Could you check a few things on this model? Use its own coordinates, in mm. Give positions to 0.01 mm unless a question says otherwise; leave off trailing zeros. Write each loop counter-clockwise with the first axis right and the second up, starting at its lowest first coordinate (ties: lowest second). Pieces come first, ordered by that corner, then holes. Notation, with made-up numbers: M 47,38.25 L 67,38.25 A20 cw 67,64.25 Z; hole C 84,72.5 d8. An arc over 180 degrees is marked long. One line per item, written item: value.
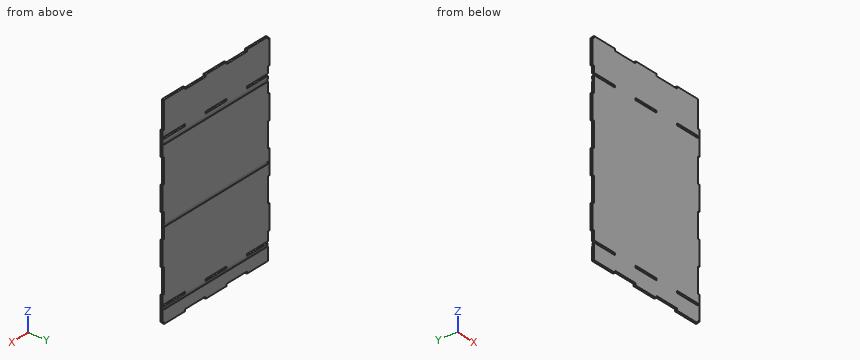
Autodesk Inventor part; units mm, degrees
ref_plane "YZ Plane" through (0, 0, 0) normal (1, 0, 0) x (0, 1, 0)
ref_plane "XZ Plane" through (0, 0, 0) normal (0, 1, 0) x (-1, 0, 0)
ref_plane "XY Plane" through (0, 0, 0) normal (0, 0, 1) x (1, 0, 0)
sketch "Sketch1" plane through (0, 0, 0) normal (0, 1, 0) x (-1, 0, 0)
  line L0 (-125, 200) -> (125, 200) construction
  line L1 (125, 200) -> (125, -200) construction
  line L2 (125, -200) -> (-125, -200) construction
  line L3 (-125, -200) -> (-125, 200) construction
  line L4 (-125, 200) -> (125, -200) construction
  line L5 (125, 200) -> (-125, -200) construction
  line L6 (125, 200) -> (75, 200) construction
  line L7 (75, 200) -> (75, 204)
  line L8 (75, 204) -> (125, 204)
  line L9 (125, 204) -> (125, 200)
  line L10 (125, 200) -> (129, 200)
  line L11 (129, 200) -> (129, 150)
  line L12 (129, 150) -> (125, 150)
  line L13 (125, 150) -> (125, 200) construction
  line L14 (-125, 200) -> (-129, 200) construction
  line L15 (-129, 200) -> (-129, 150) construction
  line L16 (-129, 150) -> (-125, 150)
  line L17 (-125, 150) -> (-125, 200)
  line L18 (125, -200) -> (75, -200) construction
  line L19 (75, -200) -> (75, -204)
  line L20 (75, -204) -> (125, -204)
  line L21 (125, -204) -> (125, -200)
  line L22 (125, 100) -> (125, 150)
  line L23 (125, 150) -> (129, 150)
  line L24 (129, 100) -> (125, 100)
  line L25 (129, 150) -> (129, 100) construction
  line L26 (-125, 100) -> (-125, 150) construction
  line L27 (-125, 150) -> (-129, 150)
  line L28 (-129, 150) -> (-129, 100)
  line L29 (-129, 100) -> (-125, 100)
  line L30 (125, 50) -> (125, 100) construction
  line L31 (125, 100) -> (129, 100)
  line L32 (129, 50) -> (125, 50)
  line L33 (129, 100) -> (129, 50)
  line L34 (-125, 50) -> (-125, 100)
  line L35 (-125, 100) -> (-129, 100)
  line L36 (-129, 100) -> (-129, 50) construction
  line L37 (-129, 50) -> (-125, 50)
  line L38 (125, 0) -> (125, 50)
  line L39 (125, 50) -> (129, 50)
  line L40 (129, 0) -> (125, 0)
  line L41 (129, 50) -> (129, 0) construction
  line L42 (-125, 0) -> (-125, 50) construction
  line L43 (-125, 50) -> (-129, 50)
  line L44 (-129, 50) -> (-129, 0)
  line L45 (-129, 0) -> (-125, 0)
  line L46 (125, -50) -> (125, 0) construction
  line L47 (125, 0) -> (129, 0)
  line L48 (129, -50) -> (125, -50)
  line L49 (129, 0) -> (129, -50)
  line L50 (-125, -50) -> (-125, 0)
  line L51 (-125, 0) -> (-129, 0)
  line L52 (-129, 0) -> (-129, -50) construction
  line L53 (-129, -50) -> (-125, -50)
  line L54 (125, -100) -> (125, -50)
  line L55 (125, -50) -> (129, -50)
  line L56 (129, -100) -> (125, -100)
  line L57 (129, -50) -> (129, -100) construction
  line L58 (-125, -100) -> (-125, -50) construction
  line L59 (-125, -50) -> (-129, -50)
  line L60 (-129, -50) -> (-129, -100)
  line L61 (-129, -100) -> (-125, -100)
  line L62 (125, -150) -> (125, -100) construction
  line L63 (125, -100) -> (129, -100)
  line L64 (129, -150) -> (125, -150)
  line L65 (129, -100) -> (129, -150)
  line L66 (-125, -150) -> (-125, -100)
  line L67 (-125, -100) -> (-129, -100)
  line L68 (-129, -100) -> (-129, -150) construction
  line L69 (-129, -150) -> (-125, -150)
  line L70 (125, -200) -> (125, -150)
  line L71 (125, -150) -> (129, -150)
  line L72 (129, -200) -> (125, -200) construction
  line L73 (129, -150) -> (129, -200) construction
  line L74 (-125, -200) -> (-125, -150) construction
  line L75 (-125, -150) -> (-129, -150)
  line L76 (-129, -150) -> (-129, -200)
  line L77 (-129, -200) -> (-125, -200)
  line L78 (75, 204) -> (75, 200)
  line L79 (25, 200) -> (25, 204)
  line L80 (25, 204) -> (75, 204) construction
  line L81 (75, 200) -> (25, 200)
  line L82 (75, -200) -> (25, -200)
  line L83 (25, -200) -> (25, -204)
  line L84 (25, -204) -> (75, -204) construction
  line L85 (75, -204) -> (75, -200)
  line L86 (25, 204) -> (25, 200)
  line L87 (-25, 200) -> (-25, 204)
  line L88 (-25, 204) -> (25, 204)
  line L89 (25, 200) -> (-25, 200) construction
  line L90 (25, -200) -> (-25, -200) construction
  line L91 (-25, -200) -> (-25, -204)
  line L92 (-25, -204) -> (25, -204)
  line L93 (25, -204) -> (25, -200)
  line L94 (-25, 204) -> (-25, 200)
  line L95 (-75, 200) -> (-75, 204)
  line L96 (-75, 204) -> (-25, 204) construction
  line L97 (-25, 200) -> (-75, 200)
  line L98 (-25, -200) -> (-75, -200)
  line L99 (-75, -200) -> (-75, -204)
  line L100 (-75, -204) -> (-25, -204) construction
  line L101 (-25, -204) -> (-25, -200)
  line L102 (-75, 204) -> (-75, 200)
  line L103 (-125, 200) -> (-125, 204)
  line L104 (-125, 204) -> (-75, 204)
  line L105 (-75, 200) -> (-125, 200) construction
  line L106 (-75, -200) -> (-125, -200) construction
  line L107 (-125, -200) -> (-125, -204)
  line L108 (-125, -204) -> (-75, -204)
  line L109 (-75, -204) -> (-75, -200)
  point P0 (0, 0)
  dimension "d0" = 250
  dimension "d1" = 400
  dimension "d2" = 50
  dimension "d3" = 4
  dimension "d4" = 4
  dimension "d5" = 50
  dimension "d6" = 4
  dimension "d7" = 50
  dimension "d8" = 50
  dimension "d9" = 4
  dimension "d12" = 50
  dimension "d19" = 50
extrude "Extrusion1" add sketch "Sketch1" along normal blind 4
sketch "Sketch3" plane through (0, 4, 0) normal (0, 1, 0) x (1, 0, 0)
  line L0 (-129, 50) -> (-129, 0)
  line L1 (-129, 25) -> (125, 25) construction
  line L2 (125, 0) -> (125, 50)
  line L3 (-129, 22.5) -> (125, 22.5)
  line L4 (125, 22.5) -> (125, 27.5)
  line L5 (125, 27.5) -> (-129, 27.5)
  line L6 (-129, 27.5) -> (-129, 22.5)
  line L7 (-129, 27.5) -> (-125, 27.5)
  line L8 (-125, 27.5) -> (-125, 22.5)
  line L9 (-125, 22.5) -> (-129, 22.5)
  line L10 (-129, 22.5) -> (-129, 27.5)
  line L11 (-25, -200) -> (-25, -204)
  line L12 (-25, -204) -> (25, -204)
  line L13 (25, -204) -> (25, -200)
  line L14 (25, -200) -> (75, -200)
  line L15 (75, -200) -> (75, -204)
  line L16 (75, -204) -> (125, -204)
  line L17 (125, -204) -> (125, -150)
  line L18 (125, -150) -> (129, -150)
  line L19 (129, -150) -> (129, -100)
  line L20 (129, -100) -> (125, -100)
  line L21 (125, -100) -> (125, -50)
  line L22 (125, -50) -> (129, -50)
  line L23 (129, -50) -> (129, 0)
  line L24 (129, 0) -> (125, 0)
  line L25 (125, 0) -> (125, 50)
  line L26 (125, 50) -> (129, 50)
  line L27 (129, 50) -> (129, 100)
  line L28 (129, 100) -> (125, 100)
  line L29 (125, 100) -> (125, 150)
  line L30 (125, 150) -> (129, 150)
  line L31 (129, 150) -> (129, 200)
  line L32 (129, 200) -> (125, 200)
  line L33 (125, 200) -> (125, 204)
  line L34 (125, 204) -> (75, 204)
  line L35 (75, 204) -> (75, 200)
  line L36 (75, 200) -> (25, 200)
  line L37 (25, 200) -> (25, 204)
  line L38 (25, 204) -> (-25, 204)
  line L39 (-25, 204) -> (-25, 200)
  line L40 (-25, 200) -> (-75, 200)
  line L41 (-75, 200) -> (-75, 204)
  line L42 (-75, 204) -> (-125, 204)
  line L43 (-125, 204) -> (-125, 150)
  line L44 (-125, 150) -> (-129, 150)
  line L45 (-129, 150) -> (-129, 100)
  line L46 (-129, 100) -> (-125, 100)
  line L47 (-125, 100) -> (-125, 50)
  line L48 (-125, 50) -> (-129, 50)
  line L49 (-129, 50) -> (-129, 0)
  line L50 (-129, 0) -> (-125, 0)
  line L51 (-125, 0) -> (-125, -50)
  line L52 (-125, -50) -> (-129, -50)
  line L53 (-129, -50) -> (-129, -100)
  line L54 (-129, -100) -> (-125, -100)
  line L55 (-125, -100) -> (-125, -150)
  line L56 (-125, -150) -> (-129, -150)
  line L57 (-129, -150) -> (-129, -200)
  line L58 (-129, -200) -> (-125, -200)
  line L59 (-125, -200) -> (-125, -204)
  line L60 (-125, -204) -> (-75, -204)
  line L61 (-75, -204) -> (-75, -200)
  line L62 (-75, -200) -> (-25, -200)
  line L63 (-125, -100) -> (-125, -150)
  line L64 (-125, -125) -> (129, -125) construction
  line L65 (129, -150) -> (129, -100)
  line L66 (-125, -127.5) -> (125, -127.5)
  line L67 (125, -127.5) -> (125, -122.5)
  line L68 (125, -122.5) -> (-125, -122.5)
  line L69 (-125, -122.5) -> (-125, -127.5)
  line L70 (-125, -127.5) -> (125, -122.5) construction
  line L71 (125, -127.5) -> (-125, -122.5) construction
  line L72 (125, 0) -> (125, 50)
  line L73 (-125, 0) -> (-125, -50)
  line L74 (129, 150) -> (129, 200)
  line L75 (129, 175) -> (-125, 175) construction
  line L76 (-125, 172.5) -> (125, 172.5)
  line L77 (125, 172.5) -> (125, 177.5)
  line L78 (125, 177.5) -> (-125, 177.5)
  line L79 (-125, 177.5) -> (-125, 172.5)
  line L80 (-125, 172.5) -> (125, 177.5) construction
  line L81 (125, 172.5) -> (-125, 177.5) construction
  line L82 (-125, 204) -> (-125, 150)
  line L83 (125, 100) -> (125, 150)
  point P0 (0, 0)
  point P1 (-125, 27.5)
  point P2 (-125, 22.5)
  point P3 (0, -125)
  point P4 (0, 175)
  dimension "d30" = 5
  dimension "d34" = 5
  dimension "d35" = 5
  dimension "d36" = 5
extrude "Extrusion2" cut sketch "Sketch3" against normal blind 1 contours L5 L2 L3 L8 | L43 L78 L77 L76 | L68 L67 L66 L55
sketch "Sketch4" plane through (0, 4, 0) normal (0, 1, 0) x (1, 0, 0)
  line L0 (-125, -133) -> (-75, -133)
  line L1 (-75, -133) -> (-75, -137)
  line L2 (-75, -137) -> (-125, -137)
  line L3 (-125, -137) -> (-125, -133)
  line L4 (-75, -200) -> (-25, -200)
  line L5 (125, -127.5) -> (-125, -127.5)
  line L6 (-75, -133) -> (-25, -133)
  line L7 (-25, -133) -> (-25, -137)
  line L8 (-25, -137) -> (-75, -137)
  line L9 (-75, -137) -> (-75, -133)
  line L10 (-25, -133) -> (25, -133)
  line L11 (25, -133) -> (25, -137)
  line L12 (25, -137) -> (-25, -137)
  line L13 (-25, -137) -> (-25, -133)
  line L14 (25, -133) -> (75, -133)
  line L15 (75, -133) -> (75, -137)
  line L16 (75, -137) -> (25, -137)
  line L17 (25, -137) -> (25, -133)
  line L18 (75, -133) -> (125, -133)
  line L19 (125, -133) -> (125, -137)
  line L20 (125, -137) -> (75, -137)
  line L21 (75, -137) -> (75, -133)
  line L22 (-125, 0) -> (-125, -50)
  line L23 (-125, 172) -> (-75, 172)
  line L24 (-75, 172) -> (-75, 168)
  line L25 (-75, 168) -> (-125, 168)
  line L26 (-125, 168) -> (-125, 172)
  line L27 (-75, 172) -> (-25, 172)
  line L28 (-25, 172) -> (-25, 168)
  line L29 (-25, 168) -> (-25, 172)
  line L30 (-25, 168) -> (-75, 168)
  line L31 (-75, 168) -> (-75, 172)
  line L32 (-25, 172) -> (25, 172)
  line L33 (25, 168) -> (-25, 168)
  line L34 (25, 172) -> (25, 168)
  line L35 (25, 168) -> (25, 172)
  line L36 (25, 172) -> (75, 172)
  line L37 (75, 172) -> (75, 168)
  line L38 (75, 168) -> (75, 172)
  line L39 (75, 172) -> (125, 172)
  line L40 (125, 172) -> (125, 168)
  line L41 (125, 168) -> (75, 168)
  line L42 (75, 168) -> (25, 168)
  point P0 (0, 0)
  point P1 (-125, -135)
  point P2 (-125, -122.5)
  point P3 (-75, -135)
  point P4 (-25, -135)
  point P5 (25, -135)
  point P6 (75, -135)
  point P7 (75, -133)
  point P8 (-25, -133)
  point P9 (-125, 170)
  point P10 (-25, 170)
  point P11 (-75, 170)
  point P12 (25, 170)
  point P13 (75, 170)
  dimension "d37" = 50
  dimension "d38" = 4
  dimension "d39" = 63
  dimension "d42" = 50
  dimension "d51" = 305
extrude "Extrusion3" cut sketch "Sketch4" against normal up to next contours L0 L1 L2 L3 | L10 L11 L12 L7 | L18 L19 L20 L15 | L23 L24 L25 L26 | L32 L34 L33 L28 | L39 L40 L41 L37
properties part number "Wall_V1"
1) I'm going to push flat-ended pins straight in: pin 1 (2 mm diameter, centred on y = 3, z = -36, fed in from +X); pin 2 (2 mm diameter, centred on y = 3, z = 27, fed in from -X); pin 3 (2 mm diameter, centred on x = -40.5, y = 1.5, fed in from +Z). Where does each tip first touch, or does it pass through?
Outcome:
pin 1: stops at x = 125
pin 2: stops at x = -125
pin 3: stops at z = 200
2) If we section it at C-C, the plane z = -83.5: Write out the boundary of the cut face in (x, y), then the cut area to 3 significant figures.
Outcome:
outline: M -125,0 L 129,0 L 129,4 L -125,4 Z
area: 1,020 mm^2
3) If we section it at B-B, the plane y = 0.8: Give the number of separate pieces and of enclosed holes in the cut face, then the cut area to 3 significant figures.
Outcome:
separate pieces: 1
enclosed holes: 4
area: 102,000 mm^2
4) Please list where these lines run through material, in increasing order: L1, parallel to Z at x = 62, y = 3.15; L2, parallel to Z at x = -91.5, y = 2.65; L3, parallel to Z at x = -105.5, y = 3.1. Write a range as from..to.
Outcome:
L1: z = -200..-177.5, -172.5..-27.5, -22.5..122.5, 127.5..200
L2: z = -204..-172, -168..133, 137..204
L3: z = -204..-177.5, -172.5..-172, -168..-27.5, -22.5..122.5, 127.5..133, 137..204
5) If we section it at A-A, the plane x = -17.5: Write out the boundary of the cut face in (y, z).
Outcome:
outline: M 0,-204 L 4,-204 L 4,-177.5 L 3,-177.5 L 3,-172.5 L 4,-172.5 L 4,-172 L 0,-172 Z; M 0,-168 L 4,-168 L 4,-27.5 L 3,-27.5 L 3,-22.5 L 4,-22.5 L 4,122.5 L 3,122.5 L 3,127.5 L 4,127.5 L 4,133 L 0,133 Z; M 0,137 L 4,137 L 4,204 L 0,204 Z
